from build123d import *

# Parameters (mm, degrees)
F0_R     = 2.6035
F0_R_2   = 2.2225
F1_DEPTH = 12.7
F2_SIZE2 = 2.54
F2_SIZE  = 10.16
F3_R     = 2.54
F4_R     = 2.54
F5_R     = 1.27


with BuildPart() as f1:
    # F0 (on Top) → F1 (new body)
    with BuildSketch(Plane.XY):
        with BuildLine():
            ThreePointArc((31.75, 11.1442627102), (0, 0), (-31.75, 11.1442627102))
            Line((-31.75, 11.1442627102), (-31.75, -39.6557372898))
            Line((-31.75, -39.6557372898), (31.75, -39.6557372898))
            Line((31.75, -39.6557372898), (31.75, 11.1442627102))
        make_face()
        with Locations((-18.4404, -30.1752)):
            Circle(F0_R, mode=Mode.SUBTRACT)
        with Locations((0, -13.0556)):
            Circle(F0_R_2, mode=Mode.SUBTRACT)
        with Locations((18.4404, -13.0556)):
            Circle(F0_R, mode=Mode.SUBTRACT)
    extrude(amount=F1_DEPTH)

    # F2
    f2_edges = [f1.edges().sort_by_distance(p)[0] for p in [
        (0, 0, 12.7),
    ]]
    f2_side = f1.faces().sort_by_distance((0, 0, 6.35))[0]
    chamfer(f2_edges, length=F2_SIZE, length2=F2_SIZE2, reference=f2_side)

    # F3
    f3_edges = [f1.edges().sort_by_distance(p)[0] for p in [
        (-31.75, 9.530934, 7.616675),
        (31.75, 9.530934, 7.616675),
    ]]
    fillet(f3_edges, radius=F3_R)

    # F4
    f4_edges = [f1.edges().sort_by_distance(p)[0] for p in [
        (-31.75, -39.655737, 6.35),
        (31.75, -39.655737, 6.35),
    ]]
    fillet(f4_edges, radius=F4_R)

    # F5
    f5_edges = [f1.edges().sort_by_distance(p)[0] for p in [
        (0, 0, 0),
    ]]
    fillet(f5_edges, radius=F5_R)


solid = f1.part
Part model, mm, in its own coordinate system. Coordinates: 2 decimals unless noted, no trailing zeros. Loops run counter-clockwise (first coordinate to the right, second up) from the corner with the lowest first, then second, coordinate; pieces in that order, holes last. Notation, with made-up numbers: (63, -30) -> (91, -30) arc R16 ccw to (91, -25) -> close; hole circle Ø11 at (1.5, 60). An arc over 180 degrees is marked (long way). Use a Markdown table: item, result. Add a question column.
Item 1: Band-saw the part on B-B on y = -14. Write the cut outline in (x, z), plus the area to 3 significant figures.
Item 2: Probe probe 1 along X at (y, z) = (6, 10); probe 2 along X at (y, z) = (-32.5, 5.25); probe 3 along Y at (x, z) = (-20, 4). List the from-to ranges inside material, lowest first.
Item 3: Band-saw the part on C-C on y = -29.5. Write the cut outline in (x, z), plus the area to 3 significant figures.
Item 4: Band-saw the part on A-A on x = 0. Write the cut outline in (y, z).
Item 5: Flat gauge pin, fed straight in: P1, Ø5, axis at x = 9.5, z = 11, coming from the +Y side. Where does the tip first touch, or does it go through?
Item 6: Band-saw the part on D-D on z = 4.25. Give the number of separate pieces and of enclosed holes in the cut face, plus the area to 3 significant figures.
Geometry says:
| question | item | result |
|---|---|---|
| 1 | outline | (-31.75, 0) -> (-2.01, 0) -> (-2.01, 12.7) -> (-31.75, 12.7) -> close; (2.01, 0) -> (16.01, 0) -> (16.01, 12.7) -> (2.01, 12.7) -> close; (20.87, 0) -> (31.75, 0) -> (31.75, 12.7) -> (20.87, 12.7) -> close |
| 1 | area | 694 mm² |
| 2 | probe 1 | -30.71 to -27.69, 27.69 to 30.71 |
| 2 | probe 2 | -31.75 to -19.61, -17.27 to 31.75 |
| 2 | probe 3 | -39.66 to -32.26, -28.09 to 3.71 |
| 3 | outline | (-31.75, 0) -> (-20.95, 0) -> (-20.95, 12.7) -> (-31.75, 12.7) -> close; (-15.93, 0) -> (31.75, 0) -> (31.75, 12.7) -> (-15.93, 12.7) -> close |
| 3 | area | 743 mm² |
| 4 | outline | (-39.66, 0) -> (-15.28, 0) -> (-15.28, 12.7) -> (-39.66, 12.7) -> close; (-10.83, 0) -> (-1.27, 0) arc R1.27 ccw to (0, 1.27) -> (0, 2.54) -> (-2.54, 12.7) -> (-10.83, 12.7) -> close |
| 5 | P1 | y = -0.45 |
| 6 | separate pieces | 1 |
| 6 | enclosed holes | 3 |
| 6 | area | 2,640 mm² |
